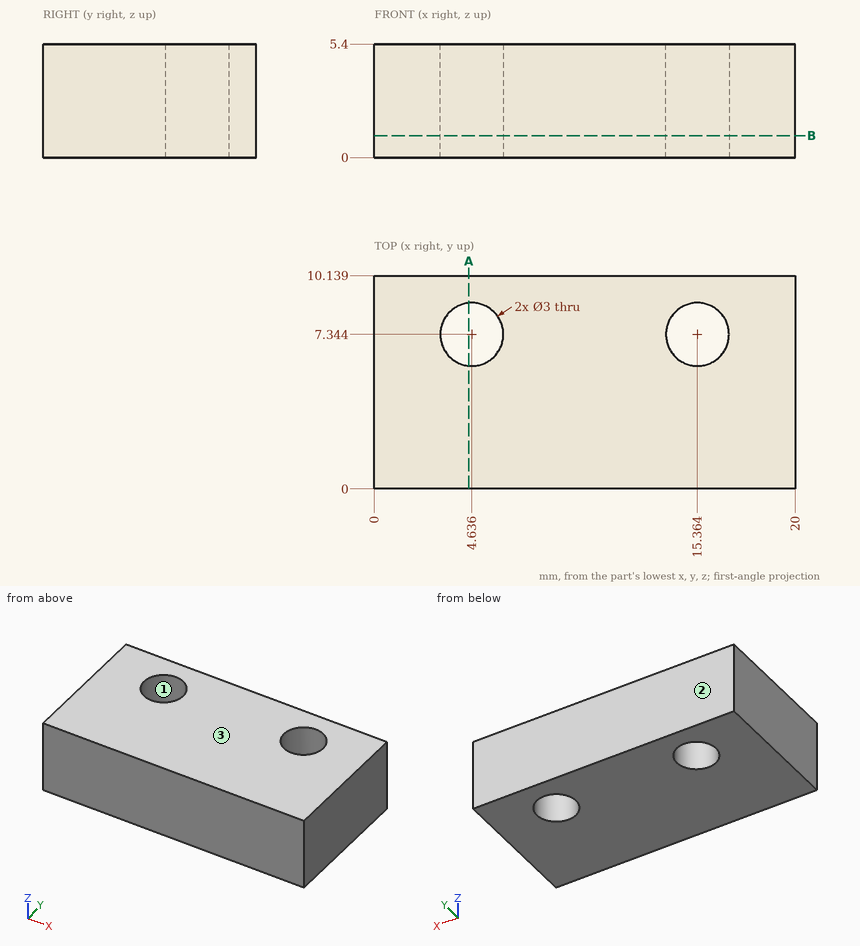
Geometry: see drawing. Coordinates: mm, zero at the bounding-box minimum. Round coordinates to 2 decimals unless told otherwise and drop trailing zeros. Loops run counter-clockwise (first coordinate to the right, second up) from the corner with the lowest first, then second, coordinate; pieces in that order, holes last. Notation, with made-up numbers: M -11.5,26 L -2.5,26 A10 ccw -2.5,41 Z; hole C 51,32.5 d9. An arc over 180 degrees is marked long. Use a Markdown table: item, result. Add a question column.
1. Ray query, line 1 along X through (y, z) = (7, 3.5) (1 decimal); line 2 along X through (y, z) = (8.5, 1.1); line 3 along Y through (x, z) = (3.5, 0.5) (1 decimal). Return the intervals inside material, ascending. Write a range as [from, to].
2. Cut plane B-B, the plane z = 1.05. Output: boundary loops of the cut face in (x, y).
3. Cut plane A-A, the plane x = 4.5. Output: boundary loops of the cut face in (y, z).
4. Pull-direction query (Y, two-part tool) for the marked faces 1, 2 and 3; classes: +Y half, -Y half, draft (parallel to the pull), parting line (faces both ways), or undercut.
Solution:
| question | item | result |
|---|---|---|
| 1 | line 1 | x = [0, 3.2], [6.1, 13.9], [16.8, 20] |
| 1 | line 2 | x = [0, 3.68], [5.59, 14.41], [16.32, 20] |
| 1 | line 3 | y = [0, 6.4], [8.3, 10.1] |
| 2 | outline | M 0,0 L 20,0 L 20,10.14 L 0,10.14 Z; hole C 4.64,7.34 d3; hole C 15.36,7.34 d3 |
| 3 | outline | M 0,0 L 5.85,0 L 5.85,5.4 L 0,5.4 Z; M 8.84,0 L 10.14,0 L 10.14,5.4 L 8.84,5.4 Z |
| 4 | face 1 | undercut |
| 4 | face 2 | +Y half |
| 4 | face 3 | draft |
